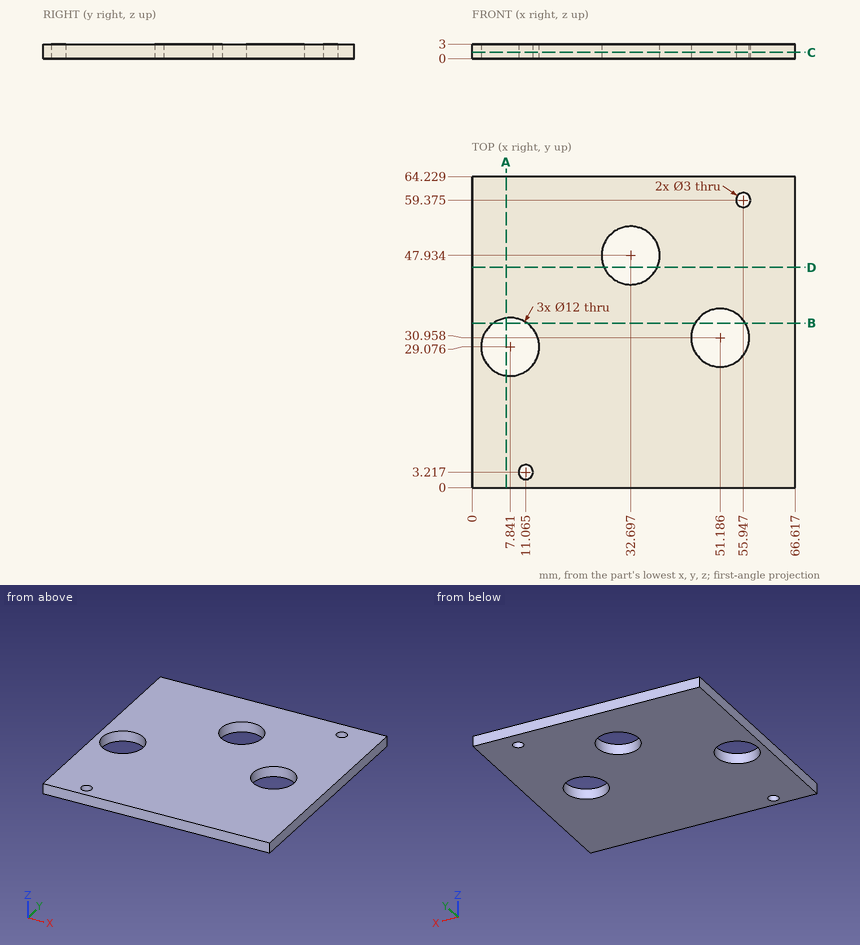
Here's the drawing with two shaded views (mm, measured from the low corner). I have some questions. Give positions to 0.01 mm unless a question says otherwise; leave off trailing zeros. Order: outer loops, then holes, each group sorted by start corner. A loop starts at its lowest first (then second) coordinate and runs counter-clockwise, first axis right, second up.
Q1. Suppose I cut it at A-A, the plane x = 7. Write out the boundary of the cut face in (y, z) (1 decimal).
Q2. Suppose I cut it at B-B, the plane y = 34. Write out the boundary of the cut face in (x, z), and give its area (3 significant figures).
Q3. If I drill on line 1 along X through (y, z) = (32, 2) (1 decimal); line 2 along X through (y, z) = (34, 1.8) (1 decimal); line 3 along Y through (x, z) = (54, 1.3) (1 decimal), over which ranges is the centre line in solid material (lowest first)?
Q4. Suppose I cut it at C-C, the plane z = 1.25. Write out the boundary of the cut face in (x, y) (1 decimal).
Q5. Suppose I cut it at D-D, the plane y = 45.5. Write out the boundary of the cut face in (x, z).
Solution:
1. outline: (0, 0) - (23.1, 0) - (23.1, 3) - (0, 3) - close; (35, 0) - (64.2, 0) - (64.2, 3) - (35, 3) - close
2. outline: (0, 0) - (4.41, 0) - (4.41, 3) - (0, 3) - close; (11.27, 0) - (46.01, 0) - (46.01, 3) - (11.27, 3) - close; (56.36, 0) - (66.62, 0) - (66.62, 3) - (56.36, 3) - close
2. area: 148 mm2
3. line 1: x = 0 to 2.6, 13.1 to 45.3, 57.1 to 66.6
3. line 2: x = 0 to 4.4, 11.3 to 46, 56.4 to 66.6
3. line 3: y = 0 to 25.7, 36.3 to 64.2
4. outline: (0, 0) - (66.6, 0) - (66.6, 64.2) - (0, 64.2) - close; hole circle Ø12 at (7.8, 29.1); hole circle Ø3 at (11.1, 3.2); hole circle Ø12 at (32.7, 47.9); hole circle Ø12 at (51.2, 31); hole circle Ø3 at (55.9, 59.4)
5. outline: (0, 0) - (27.21, 0) - (27.21, 3) - (0, 3) - close; (38.18, 0) - (66.62, 0) - (66.62, 3) - (38.18, 3) - close
